from build123d import *

# Parameters (mm, degrees)
ESQUISSE1_W       = 38
ESQUISSE1_H       = 9
ESQUISSE1_R       = 1.1
EXTRUSION1_DEPTH  = 1.4
CHANFREIN1_SIZE   = 2
ESQUISSE3_R       = 2.75
EXTRUSION2_DEPTH  = 8
D_ME1_FACE_RADIUS = 2.75
D_ME1_HEIGHT      = 3
D_ME2_FACE_RADIUS = 2.75
D_ME2_HEIGHT      = 3


# Read off the part's stored shape, not the designer's step: Dôme3
with BuildPart() as part:
    # Esquisse1 → Extrusion1 (new body)
    with BuildSketch(Plane.XY):
        with Locations((0, 12.855949766)):
            Rectangle(ESQUISSE1_W, ESQUISSE1_H)
        with Locations((16, 9.584679883)):
            Circle(ESQUISSE1_R, mode=Mode.SUBTRACT)
        with Locations((-16, 9.584679883)):
            Circle(ESQUISSE1_R, mode=Mode.SUBTRACT)
    extrude(amount=EXTRUSION1_DEPTH)

    # Chanfrein1
    chanfrein1_edges = [part.edges().sort_by_distance(p)[0] for p in [
        (-19, 17.355949766, 0.7),
        (19, 17.355949766, 0.7),
        (19, 8.355949766, 0.7),
        (-19, 8.355949766, 0.7),
    ]]
    chamfer(chanfrein1_edges, length=CHANFREIN1_SIZE)

    # Esquisse3 → Extrusion2 (add)
    with BuildSketch(Plane(origin=(0, 0, 0), x_dir=(-1, 0, 0), z_dir=(0, 0, -1))):
        with Locations((-10.007204419, 11.380286636)):
            Circle(ESQUISSE3_R)
        with Locations((-0.007204739, 11.382819166)):
            Circle(ESQUISSE3_R)
        with Locations((9.99279494, 11.385351696)):
            Circle(ESQUISSE3_R)
    extrude(amount=EXTRUSION2_DEPTH)

    # Dôme1: a dome of height H over a round flat face of radius A is a cap of a sphere of radius (A * A + H * H) / (2 * H)
    d_me1_r = (D_ME1_FACE_RADIUS * D_ME1_FACE_RADIUS + D_ME1_HEIGHT * D_ME1_HEIGHT) / (2 * D_ME1_HEIGHT)
    d_me1_base = Plane((-9.99279494, 11.385351696, -8), z_dir=(0, 0, -1))
    with Locations(d_me1_base.offset(D_ME1_HEIGHT - d_me1_r)):
        d_me1_ball = Sphere(d_me1_r, mode=Mode.PRIVATE)
    add(split(d_me1_ball, bisect_by=d_me1_base, keep=Keep.TOP, mode=Mode.PRIVATE))

    # Dôme2: a dome of height H over a round flat face of radius A is a cap of a sphere of radius (A * A + H * H) / (2 * H)
    d_me2_r = (D_ME2_FACE_RADIUS * D_ME2_FACE_RADIUS + D_ME2_HEIGHT * D_ME2_HEIGHT) / (2 * D_ME2_HEIGHT)
    d_me2_base = Plane((0.007204739, 11.382819166, -8), z_dir=(0, 0, -1))
    with Locations(d_me2_base.offset(D_ME2_HEIGHT - d_me2_r)):
        d_me2_ball = Sphere(d_me2_r, mode=Mode.PRIVATE)
    add(split(d_me2_ball, bisect_by=d_me2_base, keep=Keep.TOP, mode=Mode.PRIVATE))

    # Dôme3 outline → Dôme3 (revolve)
    with BuildSketch(Plane(origin=(10.007204419, 11.380286636, 0), x_dir=(1, 0, 0), z_dir=(0, -1, 0))):
        with BuildLine():
            Line((0, -7.999999997), (0, -11))
            ThreePointArc((0, -11), (2.034852575, -10.104864859), (2.75, -7.999999998))
            Line((2.75, -7.999999998), (0, -7.999999997))
        make_face()
    revolve(axis=Axis((10.007204419, 11.380286636, 0), (0, 0, 1)))


solid = part.part
Work out the finished part from the listing and answer in its coordinate system (mm). Round coordinates to 2 decimals unless told otherwise and drop trailing zeros. Loops run counter-clockwise (first coordinate to the right, second up) from the corner with the lowest first, then second, coordinate; pieces in that order, holes last. Notation, with made-up numbers: (68, 61.5) -> (92, 61.5) arc R30 ccw to (92, 91.5) -> close; hole circle Ø11 at (4, 66.5). An arc over 180 degrees is marked (long way). Use one line per item in the form item = value.
(1) For a pull along X with two mould halves and no side action, classify faces 1 (the flat face through (-19, 13, 1)), 2 (the flat face through (0, 8.356, 1)), 3 (the cylindrical face through (-16.873, 8.915, 0.69)), 4 (the flat face through (18.014, 16.342, 0.69)) as released by +X, released by -X, zero draft, split by the parting line, or undercut.
Answer list:
face_1 = released by -X
face_2 = zero draft
face_3 = undercut
face_4 = released by +X
(2) Find section D-D on z = -7.5. Give the vertices of the cut face in (x, y).
Answer list:
outline = circle Ø5.5 at (-9.99, 11.39); circle Ø5.5 at (0.01, 11.38); circle Ø5.5 at (10.01, 11.38)
(3) Find section B-B on y = 9.25. Give the vertices of the cut face in (x, z), then the cut area to 3 significant figures.
Answer list:
outline = (-17.89, 0) -> (-17.05, 0) -> (-17.05, 1.4) -> (-17.89, 1.4) -> close; (-14.95, 0) -> (-11.73, 0) -> (-11.73, -8) arc R1.75 ccw (long way) to (-8.26, -8) -> (-8.26, 0) -> (-1.73, 0) -> (-1.73, -8) arc R1.75 ccw (long way) to (1.74, -8) -> (1.74, 0) -> (8.27, 0) -> (8.27, -8) arc R1.76 ccw (long way) to (11.75, -8) -> (11.75, 0) -> (14.95, 0) -> (14.95, 1.4) -> (-14.95, 1.4) -> close; (17.05, 0) -> (17.89, 0) -> (17.89, 1.4) -> (17.05, 1.4) -> close
area = 145 mm2
(4) Flat-ended cylindrical pins translate along their axes: P1, Ø1, axis at x = -10, y = 9.5, coming from the -Z side; P2, Ø1, axis at x = 12, y = 14.5, coming from the -Z side; P3, Ø1, axis at x = 8, y = 13.5, coming from the -Z side. Find the tip coordinate at first contact, or state that the pin passes through.
Answer list:
P1 = -10.63
P2 = 0
P3 = -9.57
(5) Find section A-A on x = 16. Give the vertices of the cut face in (y, z).
Answer list:
outline = (8.36, 0) -> (8.48, 0) -> (8.48, 1.4) -> (8.36, 1.4) -> close; (10.68, 0) -> (17.36, 0) -> (17.36, 1.4) -> (10.68, 1.4) -> close
(6) Straight lines are drawn through the part: line 1 (X direction, y = 11, z = -0.75); line 2 (X direction, y = 9, z = 0.5); line 3 (Z direction, x = 4, y = 16.5). For each, find the intervals that lie inside material, in ascending order.
Answer list:
line_1 = -12.72 to -7.27, -2.72 to 2.73, 7.28 to 12.73
line_2 = -17.64 to -16.93, -15.07 to 15.07, 16.93 to 17.64
line_3 = 0 to 1.4
(7) Find section C-C on x = -0.5. Give the vertices of the cut face in (y, z), then the cut area to 3 significant figures.
Answer list:
outline = (8.36, 0) -> (8.68, 0) -> (8.68, -8) arc R2.71 ccw (long way) to (14.09, -8) -> (14.09, 0) -> (17.36, 0) -> (17.36, 1.4) -> (8.36, 1.4) -> close
area = 68.7 mm2
